Geometry: final body of the model. Coordinates: model frame, mm. A direction names the side the tool comes from. Give positions to 0.01 mm unless a question says otherwise; leave off trailing zeros. Write each loop counter-clockwise with the first axis right and the second up, starting at its lowest first coordinate (ties: lowest second). Pieces come first, ordered by that corner, then holes.
```python
from build123d import *


with BuildPart() as part:
    # 扫描1: sweep along a path in 草图2
    with BuildLine(Plane.XY) as sweep_1_path:
        Line((2.584252226, -4.627271381), (-136.48462728, -82.294871103))
        ThreePointArc((-136.48462728, -82.294871103), (-143.696150887, -80.251851948), (-141.653131732, -73.040328341))
        Line((-141.653131732, -73.040328341), (-2.584252226, 4.627271381))
        ThreePointArc((-2.584252226, 4.627271381), (4.627271381, 2.584252226), (2.584252226, -4.627271381))
    # 草图3 → 扫描1 (sweep)
    with BuildSketch(Plane(origin=(0, 0, 0), x_dir=(0, 0, -1), z_dir=(0.8730700718740267, 0.48759475960871657, 0))):
        Polygon((-1.535, 5.3), (1.535, 5.3), (2.990880937, 9.3), (-2.990880937, 9.3), align=None)
    sweep(path=sweep_1_path.line)


solid = part.part
```
Item 1: Reachability of faces 4 (the face through (-73.096, -30.171, -0.042)), 5 (the face through (-66.962, -45.726, -2.253)), 6 (the face through (-72.134, -31.892, 2.273)), 7 (the face through (-67.924, -44.005, 0.021)) from +Z, -Z, +X, -X, +Y, -Y: full face, straight path, thin tool, end or side. Return the list, or none.
Found:
face 4: +Z, -Z, -X, +Y
face 5: -Z
face 6: +Z
face 7: +Z, -Z
Item 2: Line query: L1, parallel to Y at x = 3, z = -0.4; L2, parallel to Y at x = -114, z = -0.05 (3 decimals); L3, parallel to X at y = -38.5, z = 0.15. Output: solid intervals per line, ascending.
Found:
L1: y = -8.98 to -4.37, 4.37 to 8.8
L2: y = -74.319 to -69.738, -57.597 to -53.015
L3: x = -88.01 to -79.81, -58.07 to -49.86
Item 3: Section C-C, the plane x = 0. Return the cut outline in (y, z) (3 decimals), plus the area to 3 significant figures.
Found:
outline: (-10.652, -2.991) - (-6.071, -1.535) - (-6.071, 1.535) - (-10.652, 2.991) - close; (5.3, -1.535) - (9.3, -2.991) - (9.3, 2.991) - (5.3, 1.535) - close
area: 38.8 mm2
Item 4: Pin query (flat end, axial travel): pin 1 Ø2 at (x, y) = (-8.5, -2) entering from +Z. Return the tip coordinate at first contact, or that it passes through.
Found:
pin 1: passes through
Item 5: Section A-A, the plane y = 0. Return the cut outline in (x, z) (3 decimals), plus the area to 3 significant figures.
Found:
outline: (-19.073, -2.991) - (-10.87, -1.535) - (-10.87, 1.535) - (-19.073, 2.991) - close; (5.3, -1.535) - (9.3, -2.991) - (9.3, 2.991) - (5.3, 1.535) - close
area: 55.2 mm2
Item 6: Pull-direction query (X, two-part tool) for faces 1 (the face through (8.02, 4.71, 0.04)), 2 (the face through (-65.973, -47.497, -0.042)), 3 (the face through (-66.935, -45.775, 2.273)); classes: +X half, -X half, draft (parallel to the pull), parting line (faces both ways), or undercut.
Found:
face 1: parting line
face 2: +X half
face 3: undercut
Item 7: Section B-B, the plane z = 0. Return the cut outline in (x, y), plus the area to 3 significant figures.
Found:
outline: (-143.6, -69.55) arc R9.3 ccw to (-134.53, -85.79) - (4.53, -8.12) arc R9.3 ccw to (-4.53, 8.12) - close; hole (-141.65, -73.04) arc R5.3 ccw to (-136.48, -82.29) - (2.58, -4.63) arc R5.3 ccw to (-2.58, 4.63) - close
area: 1,460 mm2
